from build123d import *

# Parameters (mm, degrees)
SKETCH1_R           = 2
BOSS_EXTRUDE1_DEPTH = 1


with BuildPart() as part:
    # Sketch1 → Boss-Extrude1 (new body)
    with BuildSketch(Plane(origin=(0, 0, 0), x_dir=(1, 0, 0), z_dir=(0, 1, 0))):
        with BuildLine():
            ThreePointArc((60, 7.5), (67.5, 0), (60, -7.5))
            Line((60, -7.5), (0, -7.5))
            ThreePointArc((0, -7.5), (-7.5, 0), (0, 7.5))
            Line((0, 7.5), (3, 7.5))
            Line((3, 7.5), (3, 15))
            Line((3, 15), (57, 15))
            Line((57, 15), (57, 7.5))
            Line((57, 7.5), (60, 7.5))
        make_face()
        with Locations(Location((60, 0, 0), (0, 0, 270))):
            Circle(SKETCH1_R, mode=Mode.SUBTRACT)
        with Locations(Location((0, 0, 0), (0, 0, 270))):
            Circle(SKETCH1_R, mode=Mode.SUBTRACT)
    extrude(amount=BOSS_EXTRUDE1_DEPTH)


solid = part.part
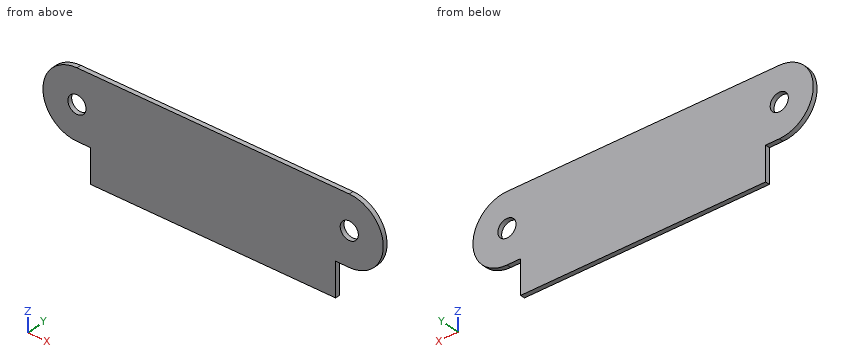
Design review of the part built by this model. Coordinates are the model's own, in mm. Round coordinates to 2 decimals unless told otherwise and drop trailing zeros. Loops run counter-clockwise (first coordinate to the right, second up) from the corner with the lowest first, then second, coordinate; pieces in that order, holes last. Notation, with made-up numbers: M 54.25,55.25 L 78.25,55.25 A10 ccw 78.25,71.25 Z; hole C 88.25,56 d9. An arc over 180 degrees is marked long. Answer as a JSON object with one key per item and string values.
Item 1: Wall thickness on L1, parallel to X at y = 0.3, z = 0; L2, parallel to X at y = 0.15, z = -9.25; L3, parallel to X at y = 0.5, z = 0.5: over which ranges is each line inside the solid? List them lowest first. Write a range as from..to.
Answer sheet:
{"L1": "x = -7.5..-2, 2..58, 62..67.5", "L2": "x = 3..57", "L3": "x = -7.48..-1.94, 1.94..58.06, 61.94..67.48"}
Item 2: Clearance check with flat-ended pins moving along their axes: P1, Ø3, axis at x = 60, z = 0, coming from the +Y side; P2, Ø0.5, axis at y = 0.5, z = -9.5, coming from the +X side. State where each tip first meets the part, or that it passes through.
Answer sheet:
{"P1": "passes through", "P2": "stops at x = 57"}
Item 3: We need section B-B on y = 0.65. Give the boundary of the cut face in (x, z).
Answer sheet:
{"outline": "M 0,-7.5 L 3,-7.5 L 3,-15 L 57,-15 L 57,-7.5 L 60,-7.5 A7.5 ccw 60,7.5 L 0,7.5 A7.5 ccw Z; hole C 0,0 d4; hole C 60,0 d4"}
Item 4: We need section A-A on z = 0. Give the boundary of the cut face in (x, y), and give its area (3 significant figures).
Answer sheet:
{"outline": "M -7.5,0 L -2,0 L -2,1 L -7.5,1 Z; M 2,0 L 58,0 L 58,1 L 2,1 Z; M 62,0 L 67.5,0 L 67.5,1 L 62,1 Z", "area": "67.0 mm^2"}
Item 5: We need section D-D on z = -4.5. Give the boundary of the cut face in (x, y).
Answer sheet:
{"outline": "M -6,0 L 66,0 L 66,1 L -6,1 Z"}
Item 6: We need section C-C on x = 1. Give the boundary of the cut face in (y, z), and give its area (3 significant figures).
Answer sheet:
{"outline": "M 0,-7.5 L 1,-7.5 L 1,-1.73 L 0,-1.73 Z; M 0,1.73 L 1,1.73 L 1,7.5 L 0,7.5 Z", "area": "11.5 mm^2"}
